The model under review builds one solid part; all positions refer to its coordinate system, in mm. Coordinates: 2 decimals unless noted, no trailing zeros. Write each loop counter-clockwise with the first axis right and the second up, starting at its lowest first coordinate (ties: lowest second). Pieces come first, ordered by that corner, then holes. Notation, with made-up numbers: (-13, -24) - (5, -24) arc R7 ccw to (5, -13) - close; hole circle Ø5 at (84.25, 81.5). An arc over 180 degrees is marked (long way). Use one line per item in the form item = value. Start each with the question number.
```python
from build123d import *

# Parameters (mm, degrees)
F0_R     = 1.5
F0_R_2   = 1.75
F1_DEPTH = 2


# Not quite as in the source:
# - a feature names something its author has since deleted; it is built from what else it names


with BuildPart() as f1:
    # F0 (on Top) → F1 (new body)
    with BuildSketch(Plane.XY):
        with BuildLine():
            Line((15.5, 28.75), (0, 28.75))
            Line((0, 28.75), (-15.5, 28.75))
            ThreePointArc((-15.5, 28.75), (-16.2071067812, 28.4571067812), (-16.5, 27.75))
            Line((-16.5, 27.75), (-16.5, 26.75))
            ThreePointArc((-16.5, 26.75), (-24.4007355432, 19.5356040873), (-26.8113935571, 9.1116960654))
            Line((-26.8113935571, 9.1116960654), (-38.0160130503, 3.886896189))
            ThreePointArc((-38.0160130503, 3.886896189), (-38.4367862343, 3.5178880103), (-38.5933947885, 2.980588402))
            Line((-38.5933947885, 2.980588402), (-38.5933947885, -2.3280322858))
            ThreePointArc((-38.5933947885, -2.3280322858), (-38.4680144957, -2.812841906), (-38.1233140528, -3.1760803819))
            Line((-38.1233140528, -3.1760803819), (-14.2431738785, -18.0980480962))
            ThreePointArc((-14.2431738785, -18.0980480962), (-13.9888919701, -18.2112616959), (-13.7132546142, -18.25))
            Line((-13.7132546142, -18.25), (0, -18.25))
            Line((0, -18.25), (13.7132546142, -18.25))
            ThreePointArc((13.7132546142, -18.25), (13.9888919701, -18.2112616959), (14.2431738785, -18.0980480962))
            Line((14.2431738785, -18.0980480962), (38.1233140528, -3.1760803819))
            ThreePointArc((38.1233140528, -3.1760803819), (38.4680144957, -2.812841906), (38.5933947885, -2.3280322858))
            Line((38.5933947885, -2.3280322858), (38.5933947885, 2.980588402))
            ThreePointArc((38.5933947885, 2.980588402), (38.4367862343, 3.5178880103), (38.0160130503, 3.886896189))
            Line((38.0160130503, 3.886896189), (26.8113935571, 9.1116960654))
            ThreePointArc((26.8113935571, 9.1116960654), (24.4007355432, 19.5356040873), (16.5, 26.75))
            Line((16.5, 26.75), (16.5, 27.75))
            ThreePointArc((16.5, 27.75), (16.2071067812, 28.4571067812), (15.5, 28.75))
        make_face()
        with Locations((-30.1321178182, -4.0957602214)):
            Circle(F0_R, mode=Mode.SUBTRACT)
        with Locations((-33, 0)):
            Circle(F0_R_2, mode=Mode.SUBTRACT)
        with Locations((30.1321178182, -4.0957602214)):
            Circle(F0_R, mode=Mode.SUBTRACT)
        with Locations((33, 0)):
            Circle(F0_R_2, mode=Mode.SUBTRACT)
    extrude(amount=F1_DEPTH)


solid = f1.part
```
1. The part is to be moulded in two halves that separate along X. For faces 1 (the flat face through (-38.593, 0, 1)), 2 (the flat face through (0, -18.25, 1)), 3 (the cylindrical face through (-28.7, -3.65, 0.99)), 4 (the flat face through (32.492, 6.463, 0.986)), say which applies: released by +X, released by -X, zero draft, split by the parting line, or undercut.
2. Take a section at B-B (x = 33). State the section outline as (y, z) points.
3. Take a section at C-C (z = 1.6). State the section outline as (x, y) points.
4. For P1, Ø1.1, axis at y = 27, z = 0.5, coming from the -X side; P2, Ø0.8, axis at y = 27.5, z = 1.5, coming from the +X side, all flat-tipped, find the tip position at first contact; note any pin that passes through.
5. Take a section at D-D (x = -23). State the section outline as (y, z) points, plus the area to 3 significant figures.
6. Take a section at A-A (y = 0). State the section outline as (x, z) points.
7. For L1, parallel to X at y = -4.5, z = 0.55; L2, parallel to Y at x = 18, z = 1.3; L3, parallel to X at y = 25.5, z = 1.5, list the stretches that pass through material, from the lowest coordinate up.
Returned:
q1.face_1 = released by -X
q1.face_2 = zero draft
q1.face_3 = undercut
q1.face_4 = released by +X
q2.outline = (-6.38, 0) - (-1.75, 0) - (-1.75, 2) - (-6.38, 2) - close; (1.75, 0) - (6.23, 0) - (6.23, 2) - (1.75, 2) - close
q3.outline = (-38.59, -2.33) arc R1 ccw to (-38.12, -3.18) - (-14.24, -18.1) arc R1 ccw to (-13.71, -18.25) - (13.71, -18.25) arc R1 ccw to (14.24, -18.1) - (38.12, -3.18) arc R1 ccw to (38.59, -2.33) - (38.59, 2.98) arc R1 ccw to (38.02, 3.89) - (26.81, 9.11) arc R18 ccw to (16.5, 26.75) - (16.5, 27.75) arc R1 ccw to (15.5, 28.75) - (-15.5, 28.75) arc R1 ccw to (-16.5, 27.75) - (-16.5, 26.75) arc R18 ccw to (-26.81, 9.11) - (-38.02, 3.89) arc R1 ccw to (-38.59, 2.98) - close; hole circle Ø3.5 at (-33, 0); hole circle Ø3 at (-30.13, -4.1); hole circle Ø3 at (30.13, -4.1); hole circle Ø3.5 at (33, 0)
q4.P1 = -17.11
q4.P2 = 16.5
q5.outline = (-12.63, 0) - (21.59, 0) - (21.59, 2) - (-12.63, 2) - close
q5.area = 68.4 mm²
q6.outline = (-38.59, 0) - (-34.75, 0) - (-34.75, 2) - (-38.59, 2) - close; (-31.25, 0) - (31.25, 0) - (31.25, 2) - (-31.25, 2) - close; (34.75, 0) - (38.59, 0) - (38.59, 2) - (34.75, 2) - close
q7.L1 = -36 to -31.58, -28.69 to 28.69, 31.58 to 36
q7.L2 = -15.75 to 25.96
q7.L3 = -18.74 to 18.74
